For this review, use the dimensioned drawing (mm, ordinates from the lowest corner) and the shaded views. A direction names the side the tool comes from. Round coordinates to 2 decimals unless told otherwise and drop trailing zeros. Loops run counter-clockwise (first coordinate to the right, second up) from the corner with the lowest first, then second, coordinate; pieces in that order, holes last. Notation, with made-up numbers: M 32,69.25 L 36,69.25 A12 cw 36,74.25 Z; hole C 29,55 d3. An arc over 180 degrees is marked long. Use a Markdown table: item, result. Add a question column.
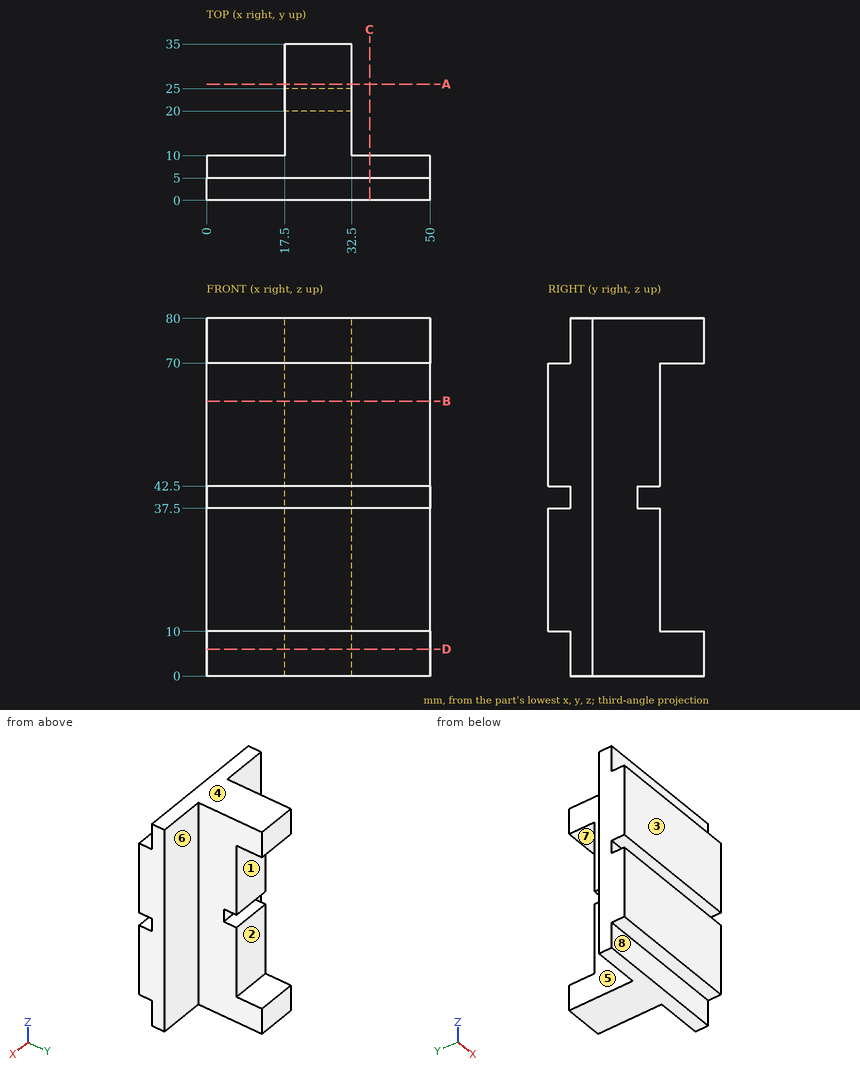
(1) Insertion check: pin 1 Ø4 at (x, y) = (36, 1.5) entering from +Z; pin 2 Ø12 at (x, z) = (31.5, 24) entering from +Y; pin 3 Ø20 at (y, z) = (26, 24) entering from -X. Each pin has a flat end and moves straight along its axis. Give the tip position at first contact, or say it passes through.
(2) Draft analysis for pull direction Z (two halves, no side actions). For the marked faces 1, 2, 3 and 4, state which applies: released by +Z, released by -Z, zero draft, split by the parting line, or undercut.
(3) Consider section A-A, the plane y = 26. Give the boundary of the cut face in (x, z), then the cut area to 3 significant figures.
(4) Consider section C-C, the plane x = 36.5. Give the boundary of the cut face in (y, z).
(5) Consider section B-B, the plane z = 61.5. Give the boundary of the cut face in (x, y).
(6) To check wall thickness, follow probe 1 along Z at (x, y) = (20.5, 2.5); probe 2 along Y at (x, z) = (25.5, 35); probe 3 along X at (y, z) = (12.5, 56.5). State the ranges of each line that lie inside material, in increasing order.
(7) For the marked faces 5, 6, 7 and 8, list the 3-axis set-ups (+Z, -Z, +X, -X, +Y, -Y) from which the entire face can be reached by the end or side of a thin tool; tool diameter is ignored.
(8) Consider section D-D, the plane z = 6. Give the boundary of the cut face in (x, y).
Found:
| question | item | result |
|---|---|---|
| 1 | pin 1 | stops at z = 70 |
| 1 | pin 2 | stops at y = 25 |
| 1 | pin 3 | stops at x = 17.5 |
| 2 | face 1 | undercut |
| 2 | face 2 | undercut |
| 2 | face 3 | zero draft |
| 2 | face 4 | released by +Z |
| 3 | outline | M 17.5,0 L 32.5,0 L 32.5,10 L 17.5,10 Z; M 17.5,70 L 32.5,70 L 32.5,80 L 17.5,80 Z |
| 3 | area | 300 mm^2 |
| 4 | outline | M 0,10 L 5,10 L 5,0 L 10,0 L 10,80 L 5,80 L 5,70 L 0,70 L 0,42.5 L 5,42.5 L 5,37.5 L 0,37.5 Z |
| 5 | outline | M 0,0 L 50,0 L 50,10 L 32.5,10 L 32.5,25 L 17.5,25 L 17.5,10 L 0,10 Z |
| 6 | probe 1 | z = 10 to 37.5, 42.5 to 70 |
| 6 | probe 2 | y = 0 to 25 |
| 6 | probe 3 | x = 17.5 to 32.5 |
| 7 | face 5 | +Z, -Z, -X, +Y |
| 7 | face 6 | +Z, -Z, +X, +Y |
| 7 | face 7 | +X, -X, +Y |
| 7 | face 8 | -Z, +X, -X, -Y |
| 8 | outline | M 0,5 L 50,5 L 50,10 L 32.5,10 L 32.5,35 L 17.5,35 L 17.5,10 L 0,10 Z |
